Read the model definition and answer for the solid it produces. Units are mm, in the model's axes. A direction names the side the tool comes from. Round coordinates to 2 decimals unless told otherwise and drop trailing zeros. Write each loop counter-clockwise with the first axis right and the second up, starting at its lowest first coordinate (ties: lowest second). Pieces come first, ordered by that corner, then holes. Notation, with made-up numbers: (-33.75, 85.25) -> (-19.75, 85.25) arc R7 cw to (-19.75, 94.25) -> close; hole circle Ø1 at (58.5, 30). An arc over 180 degrees is marked (long way). Return JSON: item names as keys, results as strings. Group by question number.
(1) A cutting plane is placed at C-C on y = -1. Give the vertices of the cut face in (x, z).
(2) For faces 1 (the cylindrical face through (18.37, -9.15, 5.53)), 2 (the cylindrical face through (-1, 0, 14)), 3 (the flat face through (30, -9, 17)), 4 (the flat face through (56, -6.5, -17)), 5 (the cylindrical face through (-19.36, -24.53, -19.73)), determine the directions among +Z, -Z, +X, -X, +Y, -Y from which every point of the face is accessible in a straight line to the end or side of a thin tool.
(3) A cutting plane is placed at A-A on x = 10.5. Give the vertices of the cut face in (y, z).
(4) Given pin 1 (11 mm diameter, centred on x = 23, z = 14.5, fed in from +Y); pin 2 (11 mm diameter, centred on x = -10.5, y = -16, fed in from +Z); pin 3 (1 mm diameter, centred on x = 33, y = -16, fed in from +Z); pin 4 (4 mm diameter, centred on y = -1.5, z = 20.5, fed in from -X), each flat-ended and moving along its own axis, determine where each tip first touches the part or whether it passes through.
(5) A cutting plane is placed at B-B on z = -1. Give the vertices of the cut face in (x, y), then the cut area to 3 significant figures.
(6) A cutting plane is placed at D-D on z = 6. Give the vertices of the cut face in (x, y).
(7) Straight lines are drawn through the part: line 1 (Z direction, x = 23, y = -5.25); line 2 (Z direction, x = 5, y = 0); line 3 (X direction, y = -18, z = -28.5). For each, find the intervals that lie inside material, in ascending order.
(8) The mould has two halves that part along X. Classify faces 6 (the flat face through (-15.8, -30.23, -26.06)), 7 (the flat face through (16, 0, 22)), 8 (the cylindrical face through (19.767, -5.486, 13.159)), 9 (the cylindrical face through (2.802, -24.485, -21.619)): released by +X, released by -X, zero draft, split by the parting line, or undercut.
```python
from build123d import *

# Parameters (mm, degrees)
BOX_W           = 34.5
BOX_H           = 16
BOX_DEPTH       = 59
SKETCH_R        = 4
POCKET_DEPTH    = 34.501
POCKET001_DEPTH = 3.5000000001
BOX001_W        = 45
BOX001_H        = 9.5
BOX001_DEPTH    = 50
SKETCH008_R     = 1.75
POCKET002_DEPTH = 9.5010000001
PAD_DEPTH       = 8
PAD001_DEPTH    = 2
SKETCH009_R     = 3.5
POCKET003_DEPTH = 2
PAD002_DEPTH    = 50
SKETCH013_R     = 6
PAD003_DEPTH    = 17
SKETCH019_W     = 9
SKETCH019_H     = 5.5
PAD004_DEPTH    = 2
SKETCH015_W     = 3
SKETCH015_H     = 4
GROOVE_ANGLE    = 40
SKETCH016_W     = 3
SKETCH016_H     = 4
POCKET004_DEPTH = 5
SKETCH020_W     = 6.4
SKETCH020_H     = 3
PAD005_DEPTH    = 8
SKETCH021_R     = 1.7
POCKET005_DEPTH = 13
POCKET006_DEPTH = 15
PAD006_DEPTH    = 17


with BuildPart() as pocket001:
    # Box → Box (new body)
    with BuildSketch(Plane(origin=(-18, -8, -30), x_dir=(1, 0, 0), z_dir=(0, 0, 1))):
        with Locations((17.25, 8)):
            Rectangle(BOX_W, BOX_H)
    extrude(amount=BOX_DEPTH)

    # Sketch → Pocket (cut, through all)
    with BuildSketch(Plane(origin=(16.5, -8, -30), x_dir=(0, 1, 0), z_dir=(1, 0, 0))):
        with Locations((8, 51)):
            Circle(SKETCH_R)
        with Locations((8, 6)):
            Circle(SKETCH_R)
        with BuildLine():
            ThreePointArc((12.5, 39.4999793754), (8.0000103123, 44), (3.5, 39.5))
            Line((3.5, 39.5), (3.5, 14.5))
            Line((3.5, 14.5), (6, 12))
            Line((6, 12), (10, 12))
            Line((10, 12), (12.5, 14.5))
            Line((12.5, 14.5), (12.5, 39.4999793754))
        make_face()
    extrude(amount=-POCKET_DEPTH, mode=Mode.SUBTRACT)

    # Sketch007 → Pocket001 (cut)
    with BuildSketch(Plane(origin=(-18, 8, -30), x_dir=(-1, 0, 0), z_dir=(0, 1, 0))):
        Polygon((-34.5, 39.4999793754), (-24.8503628945, 27.9999896877), (-24.8503628945, 25.9999896877), (-34.5, 14.5), align=None)
    extrude(amount=-POCKET001_DEPTH, mode=Mode.SUBTRACT)


with BuildPart() as pad006:
    # Box001 → Box001 (new body)
    with BuildSketch(Plane(origin=(16, -14, -30), x_dir=(1, 0, 0), z_dir=(0, 0, 1))):
        with Locations((22.5, 4.75)):
            Rectangle(BOX001_W, BOX001_H)
    extrude(amount=BOX001_DEPTH)

    # Sketch008 → Pocket002 (cut, through all)
    with BuildSketch(Plane(origin=(16, -14, -30), x_dir=(1, 0, 0), z_dir=(0, -1, 0))):
        with Locations((7, 44.5)):
            Circle(SKETCH008_R)
        with Locations((7, 13.5)):
            Circle(SKETCH008_R)
        with Locations((38, 13.5)):
            Circle(SKETCH008_R)
        Polygon((14, 50), (14, 43), (8.5, 37.5), (8.5, 21.5), (14, 16), (32.692131, 16), (32.692131, 18), (45, 18), (45, 50), align=None)
        Polygon((45, 9.1923881554), (35.8076118446, 0), (45, 0), align=None)
    extrude(amount=-POCKET002_DEPTH, mode=Mode.SUBTRACT)

    # Fusion: union Pocket001
    add(pocket001.part)

    # Sketch010 → Pad (new body)
    with BuildSketch(Plane(origin=(0, 0, -30), x_dir=(1, 0, 0), z_dir=(0, 0, -1))):
        with BuildLine():
            ThreePointArc((25.4999662688, 4.4999999999), (19.1360389694, 1.8639610307), (16.5000000001, -4.4999662687))
            Line((16.5000000001, -4.4999662687), (16.5000000001, 4.4999999999))
            Line((16.5000000001, 4.4999999999), (25.4999662688, 4.4999999999))
        make_face()
    extrude(amount=-PAD_DEPTH)

    # Sketch011 → Pad001 (new body)
    with BuildSketch(Plane.YZ.offset(16.5)):
        with BuildLine():
            ThreePointArc((-3.4641016151, -22), (0, -28), (3.4641016151, -22))
            Line((-3.4641016151, -22), (3.4641016151, -22))
        make_face()
    extrude(amount=-PAD001_DEPTH)

    # Sketch009 → Pocket003 (cut)
    with BuildSketch(Plane(origin=(0, -4.5, 0), x_dir=(-1, 0, 0), z_dir=(0, 1, 0))):
        with Locations((-23, 14.5)):
            Circle(SKETCH009_R)
        with Locations((-54, -16.5)):
            Circle(SKETCH009_R)
        with Locations((-23, -16.5)):
            Circle(SKETCH009_R)
    extrude(amount=-POCKET003_DEPTH, mode=Mode.SUBTRACT)

    # Sketch012 → Pad002 (new body)
    with BuildSketch(Plane(origin=(0, 0, -30), x_dir=(1, 0, 0), z_dir=(0, 0, -1))):
        with BuildLine():
            ThreePointArc((15.9999999999, 18.0000351724), (15.4138656704, 20.9466786767), (13.7447222151, 23.4447222151))
            Line((13.7447222151, 23.4447222151), (12.6133513652, 22.3133513652))
            ThreePointArc((11.6013945082, 23.1294048681), (4.4708258711, 13.2515870556), (12.6133513652, 22.3133513652))
            Line((11.6013945082, 23.1294048681), (12.4673340514, 24.4748225384))
            ThreePointArc((12.4673340514, 24.4748225384), (4.6120940547, 24.759389746), (0.6000000001, 18.0000351024))
            Line((0.6000000001, 18.0000351024), (0.6000000001, 8))
            Line((0.6000000001, 8), (15.9999999999, 8))
            Line((15.9999999999, 18.0000351724), (15.9999999999, 8))
        make_face()
    extrude(amount=-PAD002_DEPTH)

    # Sketch013 → Pad003 (new body)
    with BuildSketch(Plane(origin=(0, 0, -30), x_dir=(1, 0, 0), z_dir=(0, 0, -1))):
        with BuildLine():
            ThreePointArc((1.3480393737, 25.435516441), (-17.5103595019, 26.8672185857), (-16.2, 8))
            Line((-16.2, 8), (0.6000000001, 8))
            Line((0.6000000001, 8), (0.6, 18.0000060082))
            ThreePointArc((4.5689954494, 24.7356963295), (1.6660458786, 21.9090475457), (0.6, 18.0000060082))
            ThreePointArc((1.3480393737, 25.435516441), (2.8268537634, 24.4796180457), (4.5689954493, 24.7356963295))
        make_face()
        with Locations((-8.7, 18)):
            Circle(SKETCH013_R, mode=Mode.SUBTRACT)
    extrude(amount=-PAD003_DEPTH)

    # Sketch019 → Pad004 (new body)
    with BuildSketch(Plane.YZ.offset(16.5)):
        with Locations((0, 19.25)):
            Rectangle(SKETCH019_W, SKETCH019_H)
    extrude(amount=-PAD004_DEPTH)

    # Sketch015 → Groove (revolve, cut)
    with BuildSketch(Plane.XZ.offset(14)):
        with Locations((17.5, 5.5)):
            Rectangle(SKETCH015_W, SKETCH015_H)
    revolve(axis=Axis((0, -14, 0), (0, 0, 1)), revolution_arc=GROOVE_ANGLE, mode=Mode.SUBTRACT)

    # Sketch016 → Pocket004 (cut)
    with BuildSketch(Plane.XZ.offset(8)):
        with Locations((-0.8999999999, 5.5)):
            Rectangle(SKETCH016_W, SKETCH016_H)
    extrude(amount=-POCKET004_DEPTH, mode=Mode.SUBTRACT)

    # Sketch020 → Pad005 (new body)
    with BuildSketch(Plane(origin=(0, 0, -30), x_dir=(1, 0, 0), z_dir=(0, 0, -1))):
        Polygon((-19.3039162536, 24.6186826549), (-12.2, 36), (-5.2, 36), (1.3480393737, 25.435516441), align=None)
        with Locations((-8.7, 32)):
            Rectangle(SKETCH020_W, SKETCH020_H, mode=Mode.SUBTRACT)
    extrude(amount=-PAD005_DEPTH)

    # Sketch021 → Pocket005 (cut)
    with BuildSketch(Plane.XZ.offset(36)):
        with Locations((-8.7, -26)):
            Circle(SKETCH021_R)
    extrude(amount=-POCKET005_DEPTH, mode=Mode.SUBTRACT)

    # Sketch022 → Pocket006 (cut, symmetric)
    with BuildSketch(Plane.XY.offset(-13)):
        Polygon((-3.7636551984, -26.55), (1.1726896031, -18), (-3.7636551984, -9.45), (-13.6363448016, -9.45), (-18.5726896031, -18), (-13.6363448016, -26.55), align=None)
    extrude(amount=POCKET006_DEPTH, both=True, mode=Mode.SUBTRACT)

    # Sketch024 → Pad006 (new body)
    with BuildSketch(Plane(origin=(0, 0, -30), x_dir=(1, 0, 0), z_dir=(0, 0, -1))):
        Polygon((-18, 9.6477547929), (-18, 8), (-16.2, 8), align=None)
    extrude(amount=-PAD006_DEPTH)


solid = pad006.part
```
Checks:
{
 "1": {"outline": "(-18, -30) -> (18.38, -30) -> (18.38, -22) -> (14.5, -22) -> (14.5, -27.87) -> (-18, -27.87) -> close; (-18, -20.13) -> (16.5, -20.13) -> (16.5, -18) -> (-18, -18) -> close; (-18, 13.89) -> (16.5, 13.89) -> (16.5, 22) -> (14.5, 22) -> (14.5, 17.13) -> (-18, 17.13) -> close; (-18, 24.87) -> (16.5, 24.87) -> (16.5, 29) -> (-18, 29) -> close"},
 "2": {"face 1": "-Y", "face 2": "+X, -X", "face 3": "+Z, +X, +Y, -Y", "face 4": "+Y", "face 5": "+Z"},
 "3": {"outline": "(-25.38, -30) -> (-23.69, -30) -> (-23.69, 20) -> (-25.38, 20) -> close; (-12.31, -30) -> (8, -30) -> (8, -8.35) -> (4.5, -8.35) -> (4.5, -15.5) -> (2, -18) -> (-2, -18) -> (-4.5, -15.5) -> (-4.5, 9.5) arc R4.5 cw to (4.5, 9.5) -> (4.5, 2.35) -> (8, 2.35) -> (8, 29) -> (-8, 29) -> (-8, 20) -> (-12.31, 20) -> close; hole circle Ø8 at (0, -24); hole circle Ø8 at (0, 21)"},
 "4": {"pin 1": "stops at y = -4.5", "pin 2": "stops at z = -28", "pin 3": "passes through", "pin 4": "stops at x = 14.5"},
 "5": {"outline": "(-18, -8) -> (0.6, -8) -> (0.6, -17.01) -> (1.17, -18) -> (0.65, -18.9) arc R7.7 ccw to (12.47, -24.47) -> (11.6, -23.13) arc R6.1 cw (long way) to (12.61, -22.31) -> (13.74, -23.44) arc R7.7 ccw to (16, -18) -> (16, -14) -> (24.5, -14) -> (24.5, -4.5) -> (-18, -4.5) -> close; (-18, 4.5) -> (7.69, 4.5) -> (7.69, 8) -> (-18, 8) -> close", "area": "417 mm^2"},
 "6": {"outline": "(-18, -8) -> (-2.4, -8) -> (-2.4, -4.5) -> (-18, -4.5) -> close; (-18, 4.5) -> (13.56, 4.5) -> (13.56, 8) -> (-18, 8) -> close; (0.6, -18) arc R7.7 ccw to (12.47, -24.47) -> (11.6, -23.13) arc R6.1 cw (long way) to (12.61, -22.31) -> (13.74, -23.44) arc R7.7 ccw to (16, -18) -> (16, -14) arc R16 ccw to (12.87, -4.5) -> (0.6, -4.5) -> close; (16.45, -4.5) arc R19 cw to (19, -14) -> (24.5, -14) -> (24.5, -4.5) -> close"},
 "7": {"line 1": "z = -30 to -20, -13 to 11, 18 to 20", "line 2": "z = -30 to -28, -20 to -18, 14 to 17, 25 to 29", "line 3": "x = -21.2 to -14.7, -2.7 to 2.2, 14.4 to 16"},
 "8": {"face 6": "released by -X", "face 7": "zero draft", "face 8": "undercut", "face 9": "undercut"}
}
